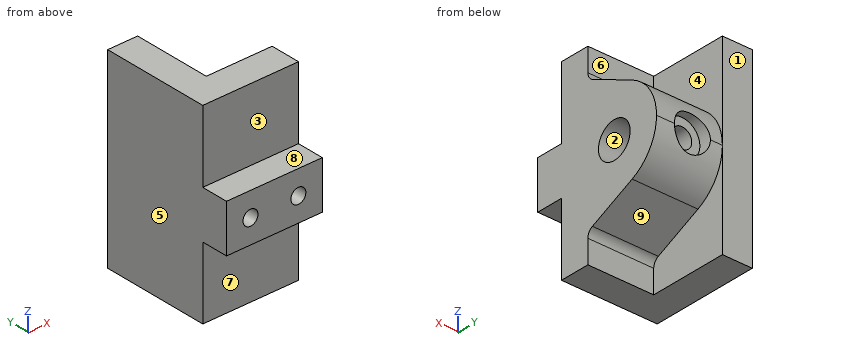
from build123d import *

# Parameters (mm, degrees)
SKETCH1_W                               = 16
SKETCH1_H                               = 9
SKETCH1_R                               = 6
BOSS_EXTRUDE1_DEPTH                     = 32
BOSS_EXTRUDE2_DEPTH                     = 10
CUT_EXTRUDE1_START                      = 32
SKETCH1_4_R                             = 6
CUT_EXTRUDE1_DEPTH                      = 24
FILLET1_R                               = 3
CBORE_START                             = 14
CBORE_FOR_M6_HEX_HEAD_BOLT1_OUTLINE_R   = 6
CBORE_FOR_M6_HEX_HEAD_BOLT1_DEPTH       = 4
CBORE_START_2                           = 7.010987826
CBORE_FOR_M6_HEX_HEAD_BOLT1_2_OUTLINE_R = 3.3
CBORE_FOR_M6_HEX_HEAD_BOLT1_2_DEPTH     = 6.989012174
M6X1_0_TAPPED_HOLE1_D                   = 5
M6X1_0_TAPPED_HOLE1_DEPTH               = 16
M6X1_0_TAPPED_HOLE1_TIP                 = 1.502151548


# Read off the part's stored shape, not the designer's step: CBORE for M6 Hex Head Bolt1
with BuildPart() as part:
    # Sketch1 → Boss-Extrude1 (new body)
    # profile 1 of 4: a face of its own
    with BuildSketch(Plane(origin=(0, 0, 0), x_dir=(0, 0, -1), z_dir=(1, 0, 0))):
        Polygon((-22.317123285, -8), (-32, -8), (-32, -18), (-8, -18), (8, -18), (32, -18), (32, -8), (22.317123285, -8), align=None)
    # profile 2 of 4: a face of its own
    with BuildSketch(Plane(origin=(0, 0, 0), x_dir=(0, 0, -1), z_dir=(1, 0, 0))):
        with Locations((0, -22.5)):
            Rectangle(SKETCH1_W, SKETCH1_H)
    # profile 3 of 4: a face of its own
    with BuildSketch(Plane(origin=(0, 0, 0), x_dir=(0, 0, -1), z_dir=(1, 0, 0))):
        with BuildLine():
            Line((-14.500924593, 8.761892188), (-22.317123285, -8))
            Line((-22.317123285, -8), (22.317123285, -8))
            Line((22.317123285, -8), (14.500924593, 8.761892188))
            ThreePointArc((14.500924593, 8.761892188), (8.596793684, 15.494263165), (-1.18e-07, 18))
            ThreePointArc((-1.18e-07, 18), (-8.596793783, 15.494263101), (-14.500924593, 8.761892188))
        make_face()
        with Locations((0, 2)):
            Circle(SKETCH1_R, mode=Mode.SUBTRACT)
    # profile 4 of 4: a face of its own
    with BuildSketch(Plane(origin=(0, 0, 0), x_dir=(0, 0, -1), z_dir=(1, 0, 0))):
        with Locations((0, 2)):
            Circle(SKETCH1_R)
    extrude(amount=BOSS_EXTRUDE1_DEPTH)

    # Sketch1<3> → Boss-Extrude2 (add)
    with BuildSketch(Plane(origin=(0, 0, 0), x_dir=(0, 0, -1), z_dir=(1, 0, 0))):
        with BuildLine():
            Line((-32, 18), (-32, -8))
            Line((-32, -8), (-22.317123285, -8))
            Line((-22.317123285, -8), (-14.500924593, 8.761892188))
            ThreePointArc((-14.500924593, 8.761892188), (-8.596793783, 15.494263101), (-1.18e-07, 18))
            Line((-1.18e-07, 18), (-32, 18))
        make_face()
        with BuildLine():
            Line((14.500924593, 8.761892188), (22.317123285, -8))
            Line((22.317123285, -8), (32, -8))
            Line((32, -8), (32, 18))
            Line((32, 18), (-1.18e-07, 18))
            ThreePointArc((-1.18e-07, 18), (8.596793684, 15.494263165), (14.500924593, 8.761892188))
        make_face()
    extrude(amount=BOSS_EXTRUDE2_DEPTH)

    # Sketch1<4> → Cut-Extrude1 (cut)
    with BuildSketch(Plane(origin=(0, 0, 0), x_dir=(0, 0, -1), z_dir=(1, 0, 0)).offset(CUT_EXTRUDE1_START)):
        with Locations((0, 2)):
            Circle(SKETCH1_4_R)
    extrude(amount=-CUT_EXTRUDE1_DEPTH, mode=Mode.SUBTRACT)

    # Fillet1
    fillet1_edges = [part.edges().sort_by_distance(p)[0] for p in [
        (21, -8, 22.317123285),
        (21, -8, -22.317123285),
    ]]
    fillet(fillet1_edges, radius=FILLET1_R)

    # CBORE for M6 Hex Head Bolt1 outline → CBORE for M6 Hex Head Bolt1 (cut)
    with BuildSketch(Plane(origin=(0, 0, 0), x_dir=(1, 0, 0), z_dir=(0, 1, 0)).offset(CBORE_START)):
        with Locations((20, 0)):
            Circle(CBORE_FOR_M6_HEX_HEAD_BOLT1_OUTLINE_R)
    extrude(amount=CBORE_FOR_M6_HEX_HEAD_BOLT1_DEPTH, mode=Mode.SUBTRACT)

    # CBORE for M6 Hex Head Bolt1 2 outline → CBORE for M6 Hex Head Bolt1 2 (cut)
    with BuildSketch(Plane(origin=(0, 0, 0), x_dir=(1, 0, 0), z_dir=(0, 1, 0)).offset(CBORE_START_2)):
        with Locations((20, 0)):
            Circle(CBORE_FOR_M6_HEX_HEAD_BOLT1_2_OUTLINE_R)
    extrude(amount=CBORE_FOR_M6_HEX_HEAD_BOLT1_2_DEPTH, mode=Mode.SUBTRACT)

    # M6x1.0 Tapped Hole1
    with Locations(Plane(origin=(0, -27, 0), x_dir=(-1, 0, 0), z_dir=(0, -1, 0))):
        with Locations((-24, 0), (-8, 0)):
            Hole(M6X1_0_TAPPED_HOLE1_D / 2, depth=M6X1_0_TAPPED_HOLE1_DEPTH)
            with Locations((0, 0, -(M6X1_0_TAPPED_HOLE1_DEPTH + M6X1_0_TAPPED_HOLE1_TIP / 2))):  # 118° drill point
                Cone(0, M6X1_0_TAPPED_HOLE1_D / 2, M6X1_0_TAPPED_HOLE1_TIP, mode=Mode.SUBTRACT)


solid = part.part
CAD build for the part. Positions are in the model's coordinates, mm. Face numbers are marked on the shaded views. A direction names the side the tool comes from. Give positions to 0.01 mm unless a question says otherwise; leave off trailing zeros. Write each loop counter-clockwise with the first axis right and the second up, starting at its lowest first coordinate (ties: lowest second). Pieces come first, ordered by that corner, then holes. Notation, with made-up numbers: (18.25, 40.25) - (49.25, 40.25) arc R21 cw to (49.25, 61.25) - close; hole circle Ø3 at (-25.75, 76.25). An arc over 180 degrees is marked (long way). Put each result on its own line as item: value.
(1) Saw through at C-C (x = 12.5). List the corners of the cut face in (y, z), then the cut area to 3 significant figures.
Working result:
outline: (-27, -8) - (-18, -8) - (-18, -32) - (-8, -32) - (-8, -24.23) arc R3 cw to (-6.27, -21.51) - (8.76, -14.5) arc R16 ccw to (8.76, 14.5) - (-6.27, 21.51) arc R3 cw to (-8, 24.23) - (-8, 32) - (-18, 32) - (-18, 8) - (-27, 8) - close; hole circle Ø12 at (2, 0)
area: 1,480 mm^2
(2) Saw through at B-B (y = 15). List the corners of the cut face in (x, z), then the cut area to 3 significant figures.
Working result:
outline: (0, -32) - (10, -32) - (10, -9.33) - (32, -9.33) - (32, 9.33) - (10, 9.33) - (10, 32) - (0, 32) - close; hole circle Ø12 at (20, 0)
area: 937 mm^2
(3) Tool access for the marked faces 5, 6, 7, 8 and 9: list every direction of +Z, -Z, +X, -X, +Y, -Y with a clear straight run to the whole face (end or side of a thin tool).
Working result:
face 5: +Z, -Z, -X, +Y, -Y
face 6: +Z, +X, +Y
face 7: -Z, +X, -X, -Y
face 8: +Z, +X, -X, -Y
face 9: -Z, +X, +Y
(4) Wall check: L1, parallel to X at y = 16, z = 0; L2, parallel to X at y = 9, z = 0; L3, parallel to X at y = -0.5, z = -1. Give the ranges that are in metal, low to high.
Working result:
L1: 0 to 14, 26 to 32
L2: 0 to 16.7, 23.3 to 32
L3: 0 to 8
(5) Saw through at D-D (z = -5). List the corners of the cut face in (x, y).
Working result:
outline: (0, -27) - (32, -27) - (32, -1.32) - (8, -1.32) - (8, 5.32) - (32, 5.32) - (32, 17.2) - (23.32, 17.2) - (23.32, 14) - (16.68, 14) - (16.68, 17.2) - (10, 17.2) - (10, 18) - (0, 18) - close
(6) Drop flat-ended pins along their axis: pin 1 Ø6 at (x, z) = (20.5, -2.5) entering from +Y; pin 2 Ø4 at (x, z) = (16, 26.5) entering from +Y; pin 3 Ø1.5 at (x, z) = (5, -16) entering from -Y. Give the stop position or say it passes through.
Working result:
pin 1: y = 14
pin 2: y = -8
pin 3: y = -18
(7) Pull direction Y, two halves, no side cores. Call the marked faces 1, 2, 3 and 4: released by +Y, released by -Y, zero draft, split by the parting line, or undercut.
Working result:
face 1: released by +Y
face 2: undercut
face 3: released by -Y
face 4: zero draft
(8) Saw through at A-A (x = 4.5). List the corners of the cut face in (y, z), then the cut area to 3 significant figures.
Working result:
outline: (-27, -8) - (-18, -8) - (-18, -32) - (18, -32) - (18, 32) - (-18, 32) - (-18, 8) - (-27, 8) - close
area: 2,450 mm^2
